Design review of the part built by this model. Coordinates are the model's own, in mm. Give positions to 0.01 mm unless a question says otherwise; leave off trailing zeros. Order: outer loops, then holes, each group sorted by start corner. A loop starts at its lowest first (then second) coordinate and runs counter-clockwise, first axis right, second up. Notation, with made-up numbers: (2.25, -39.5) -> (16.25, -39.5) arc R13 cw to (16.25, -20.5) -> close; hole circle Ø6 at (24.5, 42.5). An arc over 180 degrees is marked (long way). Return JSON: item names as keys, results as strings.
Autodesk Inventor part; units mm, degrees
ref_plane "YZ Plane" through (0, 0, 0) normal (1, 0, 0) x (0, 1, 0)
ref_plane "XZ Plane" through (0, 0, 0) normal (0, 1, 0) x (-1, 0, 0)
ref_plane "XY Plane" through (0, 0, 0) normal (0, 0, 1) x (1, 0, 0)
sketch "Sketch1" plane through (0, 0, 0) normal (0, 0, 1) x (1, 0, 0)
  line L0 (-39.1771, 0) -> (75.1229, 0)
  line L1 (75.1229, 0) -> (75.1229, -6.35)
  line L2 (75.1229, -6.35) -> (-39.1771, -6.35)
  line L3 (-39.1771, -6.35) -> (-39.1771, 0)
  point P0 (0, 0)
  dimension "d0" = 114.3
  dimension "d1" = 6.35
extrude "Extrusion1" add sketch "Sketch1" along normal blind 6.35
sketch "Sketch2" plane through (0, 0, 6.35) normal (0, 0, 1) x (1, 0, 0)
  line L0 (75.1229, 0) -> (75.1229, -6.35)
  line L1 (-39.1771, -6.35) -> (-39.1771, 0)
  line L2 (-39.1771, 0) -> (-39.1771, -3.175)
  line L3 (-39.1771, -3.175) -> (75.1229, -3.175)
  circle A0 centre (-39.1771, -3.175) radius 3.175
  circle A1 centre (75.1229, -3.175) radius 3.175
  point P0 (0, 0)
  dimension "d4" = 3.175
extrude "Extrusion2" cut sketch "Sketch2" against normal blind 6.35
sketch "Sketch3" plane through (0, 0, 6.35) normal (0, 0, 1) x (1, 0, 0)
  arc A0 (-39.1771, -6.35) -> (-39.1771, 0) centre (-39.1771, -3.175) ccw
  line L0 (75.1229, -6.35) -> (-39.1771, -6.35)
  arc A1 (75.1229, 0) -> (75.1229, -6.35) centre (75.1229, -3.175) ccw
  line L1 (-39.1771, 0) -> (75.1229, 0)
  point P0 (0, 0)
extrude "Extrusion3" cut sketch "Sketch3" against normal blind 3.175
properties part number "bar"
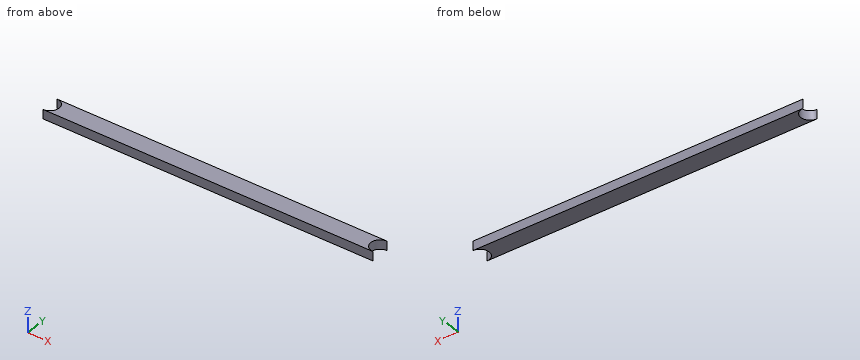
Item 1: Add section B-B (y = -1.75). Give the boundary of the cut face in (x, z) (3 decimals), plus the area to 3 significant figures.
Result set:
{"outline": "(-36.34, 0) -> (72.286, 0) -> (72.286, 3.175) -> (-36.34, 3.175) -> close", "area": "345 mm^2"}
Item 2: For pin 1 (1 mm diameter, centred on y = -5.5, z = 0.5, fed in from +X), flat-tipped, find the tip position at first contact; note if it passes through.
Result set:
{"pin 1": "stops at x = 73.67"}
Item 3: Wall thickness on L1, parallel to X at y = -3, z = 2.4; L2, parallel to X at y = -4.75, z = 1.15: over which ranges is each line inside the solid? List them lowest first. Write a range as [from, to].
Result set:
{"L1": "x = [-36.01, 71.95]", "L2": "x = [-36.42, 72.37]"}
Item 4: Add section A-A (z = 1.6). Give the boundary of the cut face in (x, y) (3 decimals), plus the area to 3 significant figures.
Result set:
{"outline": "(-39.177, -6.35) -> (75.123, -6.35) arc R3.175 cw to (75.123, 0) -> (-39.177, 0) arc R3.175 cw to start", "area": "694 mm^2"}
